Here's how the part is built. I have some questions about the finished solid (model axes, mm). Face numbers are marked on the shaded views. A direction names the side the tool comes from. Coordinates: 2 decimals unless noted, no trailing zeros. Write each loop counter-clockwise with the first axis right and the second up, starting at its lowest first coordinate (ties: lowest second). Pieces come first, ordered by that corner, then holes. Notation, with made-up numbers: (85, 32.5) -> (139, 32.5) arc R14 cw to (139, 43.5) -> close; hole circle Ø8 at (37.5, 77.5). An arc over 180 degrees is marked (long way). Use a Markdown table: item, result. Add a question column.
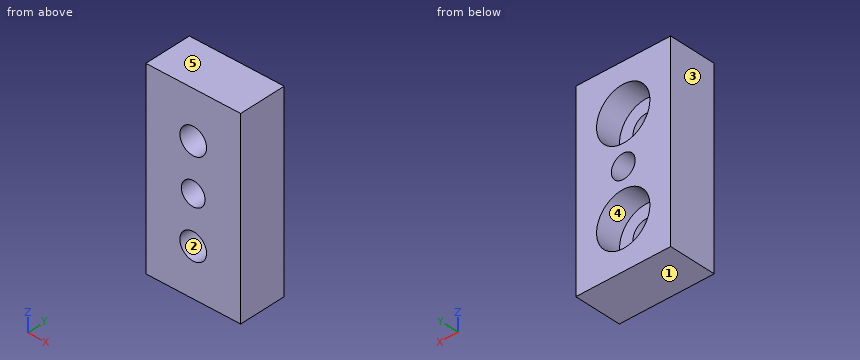
```python
from build123d import *

# Parameters (mm, degrees)
SKETCH1_W                                            = 25.4
SKETCH1_H                                            = 50.8
EXTRUDE1_DEPTH                                       = 12.7
F_1_4_0_25_DIAMETER_HOLE1_D                          = 6.35
CBORE_FOR_1_4_BINDING_HEAD_MACHINE_SCREW_D           = 7.14248
CBORE_FOR_1_4_BINDING_HEAD_MACHINE_SCREW_CBORE_D     = 14.2875
CBORE_FOR_1_4_BINDING_HEAD_MACHINE_SCREW_CBORE_DEPTH = 6.731


with BuildPart() as part:
    # Sketch1 → Extrude1 (new body)
    with BuildSketch(Plane(origin=(0, 0, 0), x_dir=(1, 0, 0), z_dir=(0, 1, 0))):
        Rectangle(SKETCH1_W, SKETCH1_H)
    extrude(amount=EXTRUDE1_DEPTH)

    # 1/4 (0.25) Diameter Hole1 (through all)
    with Locations(Plane(origin=(0, 12.7, 0), x_dir=(-1, 0, 0), z_dir=(0, 1, 0))):
        with Locations((0, 0)):
            Hole(F_1_4_0_25_DIAMETER_HOLE1_D / 2)

    # CBORE for 1/4 Binding Head Machine Screw1 (through all)
    with Locations(Plane(origin=(0, 12.7, 0), x_dir=(-1, 0, 0), z_dir=(0, 1, 0))):
        with Locations((0, -12.7), (0, 12.7)):
            CounterBoreHole(CBORE_FOR_1_4_BINDING_HEAD_MACHINE_SCREW_D / 2, CBORE_FOR_1_4_BINDING_HEAD_MACHINE_SCREW_CBORE_D / 2, CBORE_FOR_1_4_BINDING_HEAD_MACHINE_SCREW_CBORE_DEPTH)


solid = part.part
```
Q1. Which directions (+Z, -Z, +X, -X, +Y, -Y) give clear straight access to the entire face, cutting with the end or side of a thin tool? Please do the marked faces 4 and 5.
Q2. Suppose I cut it at D-D, the plane z = -12.7. Write out the boundary of the cut face in (x, y), and give its area (3 significant figures).
Q3. Suppose I cut it at C-C, the plane y = 1.5. Write out the boundary of the cut face in (x, z) (3 decimals), and give its area (3 significant figures).
Q4. Will this pin go through, and if not, where does the flat tip stop? pin 1 (2 mm diameter, centred on x = -1, z = 7.5, fed in from +Y).
Q5. Thinking about a two-plate mould opening in X: for the marked faces 1, 2 and 3, which applies, released by +X, released by -X, zero draft, split by the parting line, or undercut?
Q6. Please list where these lines run through material, in increasing order: line 1 (Z direction, x = 0, y = 9.25) (3 decimals); line 2 (Z direction, x = 0, y = 4.35) (3 decimals); line 3 (Z direction, x = -6.25, y = 7.75).
Q7. Suppose I cut it at B-B, the plane x = 0. Write out the boundary of the cut face in (y, z) (3 decimals).
Q8. Suppose I cut it at A-A, the plane z = 0. Write out the boundary of the cut face in (x, y) (3 decimals).
Answer key:
| question | item | result |
|---|---|---|
| 1 | face 4 | +Y |
| 1 | face 5 | +Z, +X, -X, +Y, -Y |
| 2 | outline | (-12.7, 0) -> (-3.57, 0) -> (-3.57, 5.97) -> (-7.14, 5.97) -> (-7.14, 12.7) -> (-12.7, 12.7) -> close; (3.57, 0) -> (12.7, 0) -> (12.7, 12.7) -> (7.14, 12.7) -> (7.14, 5.97) -> (3.57, 5.97) -> close |
| 2 | area | 184 mm^2 |
| 3 | outline | (-12.7, -25.4) -> (12.7, -25.4) -> (12.7, 25.4) -> (-12.7, 25.4) -> close; hole circle Ø7.142 at (0, -12.7); hole circle Ø7.142 at (0, 12.7); hole circle Ø6.35 at (0, 0) |
| 3 | area | 1,180 mm^2 |
| 4 | pin 1 | stops at y = 5.97 |
| 5 | face 1 | zero draft |
| 5 | face 2 | undercut |
| 5 | face 3 | released by -X |
| 6 | line 1 | z = -25.4 to -19.844, -5.556 to -3.175, 3.175 to 5.556, 19.844 to 25.4 |
| 6 | line 2 | z = -25.4 to -16.271, -9.129 to -3.175, 3.175 to 9.129, 16.271 to 25.4 |
| 6 | line 3 | z = -25.4 to -16.16, -9.24 to 9.24, 16.16 to 25.4 |
| 7 | outline | (0, -25.4) -> (12.7, -25.4) -> (12.7, -19.844) -> (5.969, -19.844) -> (5.969, -16.271) -> (0, -16.271) -> close; (0, -9.129) -> (5.969, -9.129) -> (5.969, -5.556) -> (12.7, -5.556) -> (12.7, -3.175) -> (0, -3.175) -> close; (0, 3.175) -> (12.7, 3.175) -> (12.7, 5.556) -> (5.969, 5.556) -> (5.969, 9.129) -> (0, 9.129) -> close; (0, 16.271) -> (5.969, 16.271) -> (5.969, 19.844) -> (12.7, 19.844) -> (12.7, 25.4) -> (0, 25.4) -> close |
| 8 | outline | (-12.7, 0) -> (-3.175, 0) -> (-3.175, 12.7) -> (-12.7, 12.7) -> close; (3.175, 0) -> (12.7, 0) -> (12.7, 12.7) -> (3.175, 12.7) -> close |
